from build123d import *

# Parameters (mm, degrees)
SKETCH_2_R      = 1.5
EXTRUDE_1_DEPTH = 4
FILLET_1_R      = 2


with BuildPart() as part:
    # 草图2 → 凸台-拉伸1 (new body)
    with BuildSketch(Plane.XY):
        Polygon((-14, 22.25), (14, 22.25), (14, -22.25), (-9, -22.25), (-9, 11.25), (-14, 16.25), align=None)
        with Locations((0, 7.25)):
            Circle(SKETCH_2_R, mode=Mode.SUBTRACT)
        with Locations((-1.5, 1.25)):
            Circle(SKETCH_2_R, mode=Mode.SUBTRACT)
        with Locations((6.5, 1.25)):
            Circle(SKETCH_2_R, mode=Mode.SUBTRACT)
        with Locations((-1.5, -10.75)):
            Circle(SKETCH_2_R, mode=Mode.SUBTRACT)
        with Locations((6.5, -10.75)):
            Circle(SKETCH_2_R, mode=Mode.SUBTRACT)
        with Locations((10, 7.25)):
            Circle(SKETCH_2_R, mode=Mode.SUBTRACT)
        with Locations((0, -16.75)):
            Circle(SKETCH_2_R, mode=Mode.SUBTRACT)
        with Locations((10, -16.75)):
            Circle(SKETCH_2_R, mode=Mode.SUBTRACT)
        with Locations((8, 19.25)):
            Circle(SKETCH_2_R, mode=Mode.SUBTRACT)
        with Locations((0, 19.25)):
            Circle(SKETCH_2_R, mode=Mode.SUBTRACT)
        with Locations((-8, 19.25)):
            Circle(SKETCH_2_R, mode=Mode.SUBTRACT)
    extrude(amount=EXTRUDE_1_DEPTH)

    # 圆角1
    fillet_1_edges = [part.edges().sort_by_distance(p)[0] for p in [
        (14, -22.25, 2),
        (-9, -22.25, 2),
        (-14, 22.25, 2),
        (14, 22.25, 2),
    ]]
    fillet(fillet_1_edges, radius=FILLET_1_R)


solid = part.part
Input: part model. Units: mm. Frame: model coordinates. Give positions to 0.01 mm unless a question says otherwise; leave off trailing zeros. Order: outer loops, then holes, each group sorted by start corner. A loop starts at its lowest first (then second) coordinate and runs counter-clockwise, first axis right, second up. Notation, with made-up numbers: (36.25, 79.25) - (54.25, 79.25) arc R21 ccw to (54.25, 93.25) - close; hole circle Ø1 at (42.25, -11). An arc over 180 degrees is marked (long way). Answer as a JSON object with one key per item and string values. Group by question number.
Q1. First-contact query: pin 1 Ø2.5 at (x, y) = (-8, 19.25) entering from +Z. Flat tip, straight axial feed; report the tip coordinate or a pass-through.
Q2. Cut plane C-C, the plane y = 1.25. Output: boundary loops of the cut face in (x, z).
Q3. Mould query, pull axis X, two halves, no side actions, for faces 1 (the face through (-13.4, 21.68, 2.03)), 2 (the face through (3, 0, 0)), 3 (the face through (-2.61, 2.26, 1.97)). Classes: pulls with the +X half, pulls with the -X half, needs draft (parallel to the pull), parting line crosses it, or undercut.
Q4. Line query: probe 1 along X at (y, z) = (8.5, 0.3); probe 2 along X at (y, z) = (-13.5, 2); probe 3 along X at (y, z) = (-16, 2.2). Output: solid intervals per line, ascending.
Q5. Cut plane B-B, the plane x = 10. Output: boundary loops of the cut face in (y, z), then the cut area to 3 significant figures.
Q6. Cut plane A-A, the plane y = 19.25. Output: boundary loops of the cut face in (x, z).
Q7. Cut plane D-D, the plane z = 0.8. Count the separate pieces of the cut face and the enclosed holes in it, then the cut area to 3 significant figures.
Results:
{
 "1": {"pin 1": "through"},
 "2": {"outline": "(-9, 0) - (-3, 0) - (-3, 4) - (-9, 4) - close; (0, 0) - (5, 0) - (5, 4) - (0, 4) - close; (8, 0) - (14, 0) - (14, 4) - (8, 4) - close"},
 "3": {"face 1": "pulls with the -X half", "face 2": "needs draft", "face 3": "undercut"},
 "4": {"probe 1": "-9 to -0.83, 0.83 to 9.17, 10.83 to 14", "probe 2": "-9 to 14", "probe 3": "-9 to -1.3, 1.3 to 8.7, 11.3 to 14"},
 "5": {"outline": "(-22.25, 0) - (-18.25, 0) - (-18.25, 4) - (-22.25, 4) - close; (-15.25, 0) - (5.75, 0) - (5.75, 4) - (-15.25, 4) - close; (8.75, 0) - (22.25, 0) - (22.25, 4) - (8.75, 4) - close", "area": "154 mm^2"},
 "6": {"outline": "(-14, 0) - (-9.5, 0) - (-9.5, 4) - (-14, 4) - close; (-6.5, 0) - (-1.5, 0) - (-1.5, 4) - (-6.5, 4) - close; (1.5, 0) - (6.5, 0) - (6.5, 4) - (1.5, 4) - close; (9.5, 0) - (14, 0) - (14, 4) - (9.5, 4) - close"},
 "7": {"separate pieces": "1", "enclosed holes": "11", "area": "985 mm^2"}
}
